```python
from build123d import *

# Parameters (mm, degrees)
BOSS_EXTRUDE1_DEPTH = 4
CUT_EXTRUDE3_START  = -10
CUT_EXTRUDE3_DEPTH  = 10
CUT_EXTRUDE4_DEPTH  = 10
FILLET4_START       = -1
FILLET4_DEPTH       = 6
SKETCH7_RX          = 1.83432271
SKETCH7_RY          = 1.648181576
BOSS_EXTRUDE2_DEPTH = 3
SKETCH8_R           = 1.941403724
BOSS_EXTRUDE3_DEPTH = 0.5
CUT_EXTRUDE5_DEPTH  = 5
CUT_EXTRUDE6_DEPTH  = 10


with BuildPart() as part:
    # Sketch1 → Boss-Extrude1 (new body)
    with BuildSketch(Plane(origin=(0, 0, 0), x_dir=(0, 0, -1), z_dir=(1, 0, 0))):
        with BuildLine():
            Line((6.442518848, 0), (13.409619329, 0))
            ThreePointArc((13.409619329, 0), (16.945153235, -1.464466094), (18.409619329, -5))
            Line((18.409619329, -5), (18.409619329, -20.34540211))
            ThreePointArc((18.409619329, -20.34540211), (16.945153235, -23.880936016), (13.409619329, -25.34540211))
            Line((13.409619329, -25.34540211), (6.442518848, -25.34540211))
            ThreePointArc((6.442518848, -25.34540211), (2.906984942, -23.880936016), (1.442518848, -20.34540211))
            Line((1.442518848, -20.34540211), (1.442518848, -5))
            ThreePointArc((1.442518848, -5), (2.906984942, -1.464466094), (6.442518848, 0))
        make_face()
    extrude(amount=BOSS_EXTRUDE1_DEPTH)

    # Sketch2 → Cut-Extrude3 (cut)
    with BuildSketch(Plane(origin=(4, 0, 0), x_dir=(0, 0, -1), z_dir=(1, 0, 0)).offset(CUT_EXTRUDE3_START)):
        with BuildLine():
            add(Edge.make_bspline(
                [(2.42884403, -23.286077848), (2.370716158, -22.573896831), (4.185530255, -21.12926271), (4.874517164, -17.962112227), (7.118988975, -13.802662727), (6.544049448, -7.530329658), (1.569055746, -5.349803368), (1.58046752, -3.833613753)],
                knots=[0.531334438, 0.531334438, 0.531334438, 0.531334438, 0.570400737, 0.608236932, 0.680812242, 0.778589658, 0.857107486, 0.857107486, 0.857107486, 0.857107486], degree=3))
            ThreePointArc((1.58046752, -3.833613753), (1.47712578, -4.412742239), (1.442518848, -5))
            Line((1.442518848, -5), (1.442518848, -20.34540211))
            ThreePointArc((1.442518848, -20.34540211), (1.683757797, -21.87974016), (2.384196149, -23.266021372))
            add(Edge.make_bspline(
                [(2.384196149, -23.266021372), (2.399070873, -23.272759012), (2.413953527, -23.279444568), (2.428844038, -23.286077844)],
                knots=[0.998981394, 0.998981394, 0.998981394, 0.998981394, 0.999513034, 0.999513034, 0.999513034, 0.999513034], degree=3))
        make_face()
        with BuildLine():
            Line((13.409619329, 0), (9.46398266, 0))
            add(Edge.make_bspline(
                [(9.46398266, 0), (11.207503001, -0.168664697), (14.40943711, -0.885845558), (18.093070912, -5.600973008), (14.034927819, -11.50687924), (8.23474836, -15.211494887), (7.662204752, -25.591568315), (4.542739971, -24.937885151)],
                knots=[0, 0, 0, 0, 0.077946221, 0.143334379, 0.228662798, 0.345497184, 0.490655992, 0.490655992, 0.490655992, 0.490655992], degree=3))
            add(Edge.make_bspline(
                [(4.54273997, -24.937885153), (5.749127141, -25.532851997), (7.208451258, -25.09277451), (8.521498661, -25.334156754), (8.57622256, -25.34540211)],
                knots=[0.001400322, 0.001400322, 0.001400322, 0.001400322, 0.038459748, 0.040079073, 0.040079073, 0.040079073, 0.040079073], degree=3))
            Line((8.57622256, -25.34540211), (13.409619329, -25.34540211))
            ThreePointArc((13.409619329, -25.34540211), (16.945153235, -23.880936016), (18.409619329, -20.34540211))
            Line((18.409619329, -20.34540211), (18.409619329, -5))
            ThreePointArc((18.409619329, -5), (16.945153235, -1.464466094), (13.409619329, 0))
        make_face()
        with BuildLine():
            ThreePointArc((2.906984942, -1.464466094), (4.529101686, -0.380602337), (6.442518848, 0))
            add(Edge.make_bspline(
                [(6.442518848, 0), (7.443592251, 0.121124965), (8.454170968, 0.097687179), (9.46398266, 0)],
                knots=[0.954855127, 0.954855127, 0.954855127, 0.954855127, 1, 1, 1, 1], degree=3))
            Line((9.46398266, 0), (13.409619329, 0))
            ThreePointArc((13.409619329, 0), (16.945153235, -1.464466094), (18.409619329, -5))
            Line((18.409619329, -5), (18.409619329, -20.34540211))
            ThreePointArc((18.409619329, -20.34540211), (16.945153235, -23.880936016), (13.409619329, -25.34540211))
            Line((13.409619329, -25.34540211), (8.57622256, -25.34540211))
            add(Edge.make_bspline(
                [(8.57622256, -25.34540211), (10.509849295, -25.742748085), (21.004932545, -37.507061135), (40.108036136, 7.046689321), (11.067178354, 5.045725954), (-13.182357735, 4.105959789), (-4.736766595, -20.04051671), (2.384196149, -23.266021372)],
                knots=[0.040079073, 0.040079073, 0.040079073, 0.040079073, 0.09729665, 0.409886449, 0.593670055, 0.744469586, 0.998981394, 0.998981394, 0.998981394, 0.998981394], degree=3))
            ThreePointArc((2.384196149, -23.266021372), (1.683757797, -21.87974016), (1.442518848, -20.34540211))
            Line((1.442518848, -20.34540211), (1.442518848, -5))
            ThreePointArc((1.442518848, -5), (1.47712578, -4.412742239), (1.58046752, -3.833613753))
            add(Edge.make_bspline(
                [(1.58046752, -3.833613753), (1.586363874, -3.050213083), (2.186842654, -2.121305338), (2.906984942, -1.464466094)],
                knots=[0.857107486, 0.857107486, 0.857107486, 0.857107486, 0.897676897, 0.897676897, 0.897676897, 0.897676897], degree=3))
        make_face()
    extrude(amount=CUT_EXTRUDE3_DEPTH, mode=Mode.SUBTRACT)

    # Sketch6 → Cut-Extrude4 (cut)
    with BuildSketch(Plane(origin=(4, 0, 0), x_dir=(0, 0, -1), z_dir=(1, 0, 0))):
        with BuildLine():
            add(Edge.make_bspline(
                [(6.876629539, -24.646378986), (6.348652857, -24.697603605), (5.705170416, -25.181041107), (2.967179599, -24.643973727), (6.798679283, -26.524715176), (10.198220508, -25.437781208), (7.742791771, -24.562343399), (6.876629539, -24.646378986)],
                knots=[0, 0, 0, 0, 0.142115473, 0.262842986, 0.576183637, 0.76685513, 1, 1, 1, 1], degree=3))
        make_face()
    extrude(amount=-CUT_EXTRUDE4_DEPTH, mode=Mode.SUBTRACT)

    # Fillet4: read off the stored shape, not the designer's step
    # Fillet4 outline → Fillet4 (cut)
    with BuildSketch(Plane.YZ.offset(FILLET4_START)):
        with BuildLine():
            ThreePointArc((0, -8.890200058), (-0.027061887, -9.625390775), (-0.108101078, -10.356602363))
            add(Edge.make_bspline(
                [(0, -9.46398266), (-0.028832047, -9.762025236), (-0.064132076, -10.060000995), (-0.108101078, -10.356602363)],
                knots=[0, 0, 0, 0, 0.01332436, 0.01332436, 0.01332436, 0.01332436], degree=3))
            Line((0, -9.46398266), (0, -8.890200058))
        make_face()
    extrude(amount=FILLET4_DEPTH, mode=Mode.SUBTRACT)

    # Sketch7 → Boss-Extrude2 (add)
    with BuildSketch(Plane.ZY):
        with Locations(Location((-12.079238976, -5.176946967), (0, 0, 66.52385958))):
            Ellipse(SKETCH7_RX, SKETCH7_RY)
    extrude(amount=BOSS_EXTRUDE2_DEPTH)

    # Sketch8 → Boss-Extrude3 (add)
    with BuildSketch(Plane.ZY.offset(3)):
        with Locations((-12.079238976, -5.176946967)):
            Circle(SKETCH8_R)
    extrude(amount=BOSS_EXTRUDE3_DEPTH)

    # Dome1: read off the stored shape, not the designer's step
    # Dome1 outline → Dome1 (revolve)
    with BuildSketch(Plane(origin=(0, -5.176946967, -12.079238976), x_dir=(0, 1, 0), z_dir=(0, 0, -1))):
        with BuildLine():
            Line((0, -3.499999998), (0, -8.5))
            ThreePointArc((0, -8.5), (2.681839314, -6.664401723), (1.941403723, -3.499999999))
            Line((1.941403723, -3.499999999), (0, -3.499999998))
        make_face()
    revolve(axis=Axis((0, -5.176946967, -12.079238976), (1, 0, 0)))

    # Sketch9 → Cut-Extrude5 (cut)
    with BuildSketch(Plane.ZY):
        with BuildLine():
            Line((-4.325838527, -20.140987675), (-2.486204677, -24.505449301))
            add(Edge.make_bspline(
                [(-2.486204677, -24.505449301), (3.73593799, -24.171685926), (-2.121854058, -16.126748366), (-4.325838527, -20.140987675)],
                knots=[0, 0, 0, 0, 1, 1, 1, 1], degree=3))
        make_face()
    extrude(amount=-CUT_EXTRUDE5_DEPTH, mode=Mode.SUBTRACT)

    # Sketch10 → Cut-Extrude6 (cut)
    with BuildSketch(Plane.ZY):
        with BuildLine():
            add(Edge.make_bspline(
                [(-20.598699556, -6.394321891), (-16.755827274, 0.910133144), (9.164509457, 10.912523184), (-0.036389797, -25.461480915), (-14.467778879, -53.72221039), (-27.813040504, -20.107197366), (-20.598699556, -6.394321891)],
                knots=[0, 0, 0, 0, 0.192062033, 0.555519923, 0.639436107, 1, 1, 1, 1], degree=3))
        make_face()
    extrude(amount=-CUT_EXTRUDE6_DEPTH, mode=Mode.SUBTRACT)


solid = part.part
```
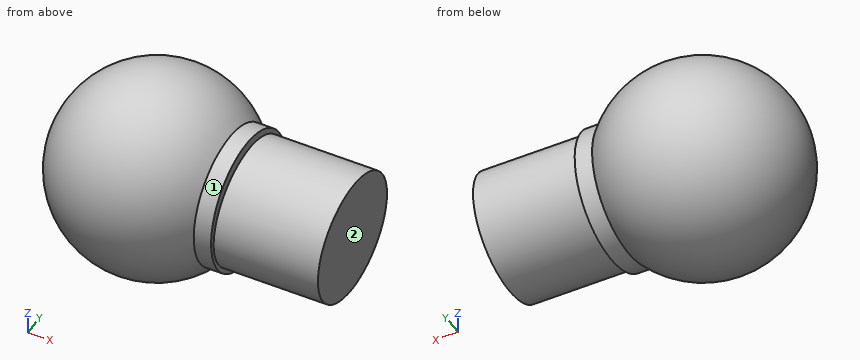
Could you check a few things on this model? Use its own coordinates, in mm. Face numbers are marked on the shaded views. A direction names the side the tool comes from. Give positions to 0.01 mm unless a question says otherwise; leave off trailing zeros. Order: outer loops, then holes, each group sorted by start corner. A loop starts at its lowest first (then second) coordinate and runs counter-clockwise, first axis right, second up.
Q1. Suppose I cut it at A-A, the plane x = -4.25. Write out the boundary of the cut face in (y, z), and give its area (3 significant figures).
Q2. For the marked faces 1 and 2, which set-ups out of +Z, -Z, +X, -X, +Y, -Y let a thin tool reach every point of the face, with its end or its side?
Q3. Suppose I cut it at B-B, the plane z = -9.9. Write out the boundary of the cut face in (x, y).
Q4. I'm going to push flat-ended pins straight in: P1, Ø1, axis at x = -7.5, z = -10.5, coming from the -Y side; P2, Ø2, axis at y = -5, z = -12, coming from the +X side; P3, Ø1, axis at y = -7, z = -10.5, coming from the -X side; P4, Ø1.5, axis at y = -5, z = -10.5, coming from the -X side. Where does each tip first touch, or does it pass through?
Q5. If I drill on line 1 along X through (y, z) = (-6.9, -14.1); line 2 along X through (y, z) = (-4.85, -11.3); line 3 along Z through (x, y) = (-5, -5.35), over which ranges is the centre line in solid material (lowest first)?
Solution:
1. outline: circle Ø5.06 at (-5.18, -12.08)
1. area: 20.1 mm2
2. face 1: +X
2. face 2: +Z, -Z, +X, +Y, -Y
3. outline: circle Ø3.76 at (-5.62, -5.18)
4. P1: stops at y = -7.29
4. P2: stops at x = 0
4. P3: stops at x = -7.77
4. P4: stops at x = -8.37
5. line 1: x = -6.73 to -4.52
5. line 2: x = -8.37 to 0
5. line 3: z = -14.88 to -9.28
